```python
from build123d import *

# Parameters (mm, degrees)
SKETCH1_W                = 19.05
SKETCH1_H                = 17.4
BOSS_EXTRUDE1_DEPTH      = 6.35
M4_CLEARANCE_HOLE1_D     = 4.5
M4_CLEARANCE_HOLE1_DEPTH = 12.7
M4_CLEARANCE_HOLE1_TIP   = 1.351936393
SKETCH4_R                = 1
CUT_EXTRUDE1_DEPTH       = 27.570378243


with BuildPart() as part:
    # Sketch1 → Boss-Extrude1 (new body)
    with BuildSketch(Plane.XY):
        with Locations((9.525, 8.7)):
            Rectangle(SKETCH1_W, SKETCH1_H)
    extrude(amount=BOSS_EXTRUDE1_DEPTH)

    # M4 Clearance Hole1
    with Locations(Plane.XY.offset(6.35)):
        with Locations((14.2875, 8.7)):
            Hole(M4_CLEARANCE_HOLE1_D / 2, depth=M4_CLEARANCE_HOLE1_DEPTH)
            with Locations((0, 0, -(M4_CLEARANCE_HOLE1_DEPTH + M4_CLEARANCE_HOLE1_TIP / 2))):  # 118° drill point
                Cone(0, M4_CLEARANCE_HOLE1_D / 2, M4_CLEARANCE_HOLE1_TIP, mode=Mode.SUBTRACT)

    # Sketch4 → Cut-Extrude1 (cut, through all)
    with BuildSketch(Plane.XY.offset(6.35)):
        with Locations((3.175, 14.225)):
            Circle(SKETCH4_R)
    extrude(amount=-CUT_EXTRUDE1_DEPTH, mode=Mode.SUBTRACT)


solid = part.part
```
CAD build for the part. Positions are in the model's coordinates, mm. Round coordinates to 2 decimals unless told otherwise and drop trailing zeros. Order: outer loops, then holes, each group sorted by start corner. A loop starts at its lowest first (then second) coordinate and runs counter-clockwise, first axis right, second up.
Item 1: Probe line 1 along Y through (x, z) = (13, 2.25); line 2 along X through (y, z) = (10, 5.25); line 3 along Y through (x, z) = (16, 0.5). List the from-to ranges inside material, lowest first.
Item 2: Saw through at B-B on x = 13.5. Write the cut outline in (y, z).
Item 3: Saw through at A-A on y = 8.7. Write the cut outline in (x, z).
Item 4: Saw through at C-C on z = 1.25. State how many separate pieces and enclosed holes the cut face has, then the cut area to 3 significant figures.
Item 5: Mould opens along X. For faces 1 (the face through (9, 9, 6.35)), 2 (the face through (2.96, 13.25, 3.22)), 3 (the face through (0, 9, 3)) say: pulls with the +X half, pulls with the -X half, needs draft (parallel to the pull), parting line crosses it, or undercut.
Reported:
1. line 1: y = 0 to 6.85, 10.55 to 17.4
1. line 2: x = 0 to 12.45, 16.12 to 19.05
1. line 3: y = 0 to 7.24, 10.16 to 17.4
2. outline: (0, 0) - (6.59, 0) - (6.59, 6.35) - (0, 6.35) - close; (10.81, 0) - (17.4, 0) - (17.4, 6.35) - (10.81, 6.35) - close
3. outline: (0, 0) - (12.04, 0) - (12.04, 6.35) - (0, 6.35) - close; (16.54, 0) - (19.05, 0) - (19.05, 6.35) - (16.54, 6.35) - close
4. separate pieces: 1
4. enclosed holes: 2
4. area: 312 mm2
5. face 1: needs draft
5. face 2: undercut
5. face 3: pulls with the -X half
